from build123d import *

# Parameters (mm, degrees)
SKETCH1_W           = 50.8
SKETCH1_H           = 50.8
BOSS_EXTRUDE1_DEPTH = 25.4
SKETCH2_W           = 25.4
SKETCH2_H           = 25.4
BOSS_EXTRUDE2_DEPTH = 25.4
SKETCH3_W           = 25.4
SKETCH3_H           = 25.4
BOSS_EXTRUDE3_DEPTH = 25.4


with BuildPart() as part:
    # Sketch1 → Boss-Extrude1 (new body)
    with BuildSketch(Plane(origin=(0, 0, 0), x_dir=(1, 0, 0), z_dir=(0, 1, 0))):
        with Locations((25.4, -25.4)):
            Rectangle(SKETCH1_W, SKETCH1_H)
    extrude(amount=BOSS_EXTRUDE1_DEPTH)

    # Sketch2 → Boss-Extrude2 (add)
    with BuildSketch(Plane(origin=(0, 25.4, 0), x_dir=(1, 0, 0), z_dir=(0, 1, 0))):
        with Locations((38.1, -38.1)):
            Rectangle(SKETCH2_W, SKETCH2_H)
    extrude(amount=BOSS_EXTRUDE2_DEPTH)

    # Sketch3 → Boss-Extrude3 (add)
    with BuildSketch(Plane.ZY.offset(-25.4)):
        with Locations((38.1, 38.1)):
            Rectangle(SKETCH3_W, SKETCH3_H)
    extrude(amount=BOSS_EXTRUDE3_DEPTH)


solid = part.part
Check sheet for the modelled part. Datum: model origin and axes. Units: mm. A direction names the side the tool comes from. Give positions to 0.01 mm unless a question says otherwise; leave off trailing zeros. Write each loop counter-clockwise with the first axis right and the second up, starting at its lowest first coordinate (ties: lowest second). Pieces come first, ordered by that corner, then holes. Notation, with made-up numbers: (72.5, 53) -> (95.5, 53) arc R17 ccw to (95.5, 69) -> close; hole circle Ø1 at (-37, 72). An arc over 180 degrees is marked (long way). One line per item, written item: value. Start each with the question number.
Item 1: Gauge pin test, flat ends, axial feed: pin 1 (12.5 mm diameter, centred on x = 36.5, z = 8, fed in from +Y); pin 2 (3 mm diameter, centred on x = 10.5, y = 40, fed in from -Z). Record the tip position at first contact, or that the pin passes through.
Item 2: Section check B-B on x = 45.5. Record the cut outline in (y, z), then the cut area to 3 significant figures.
Item 3: Material ranges on probe 1 along Y at (x, z) = (7, 6); probe 2 along Z at (x, y) = (5, 48.5), recorded low to high. Write a range as from..to.
Item 4: Section check C-C on z = 8. Record the cut outline in (x, y).
Item 5: Tool access check on faces 1 (the flat face through (50.8, 19, 31)), 2 (the flat face through (26, 38, 25.4)). Record the directions out of +Z, -Z, +X, -X, +Y, -Y that give a thin tool (end or side, any length) a straight path to the whole face; none if there is none.
Item 6: Section check A-A on y = 34.5. Record the cut outline in (x, z).
Results list:
1. pin 1: y = 25.4
1. pin 2: z = 25.4
2. outline: (0, 0) -> (25.4, 0) -> (25.4, 25.4) -> (50.8, 25.4) -> (50.8, 50.8) -> (0, 50.8) -> close
2. area: 1,940 mm²
3. probe 1: 0..25.4
3. probe 2: 25.4..50.8
4. outline: (0, 0) -> (50.8, 0) -> (50.8, 25.4) -> (0, 25.4) -> close
5. face 1: +Z, -Z, +X, +Y, -Y
5. face 2: -Z, +X, -X, +Y
6. outline: (0, 25.4) -> (50.8, 25.4) -> (50.8, 50.8) -> (0, 50.8) -> close
